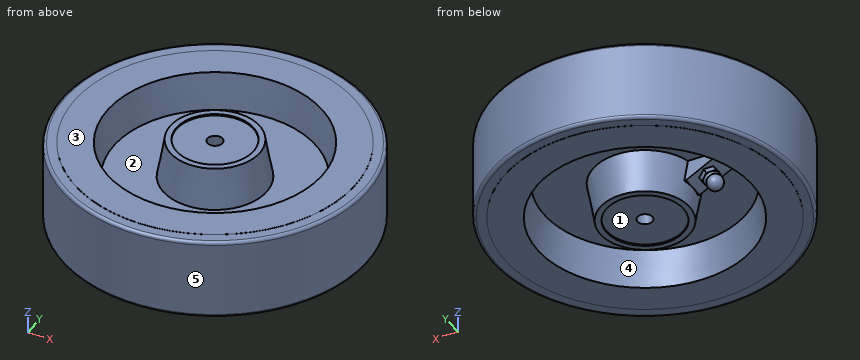
```python
from build123d import *

# Parameters (mm, degrees)
SKETCH1_R           = 150
SKETCH1_R_2         = 138
BOSS_EXTRUDE1_DEPTH = 40
FILLET4_R           = 3
BOSS_EXTRUDE2_DEPTH = 12.5
BOSS_EXTRUDE3_DEPTH = 5.5
SKETCH6_R           = 8.061337792
BOSS_EXTRUDE4_DEPTH = 3
BOSS_EXTRUDE4_TAPER = 30
SKETCH8_R           = 7.5
CUT_EXTRUDE1_DEPTH  = 229.714341483


with BuildPart() as part:
    # Sketch1 → Boss-Extrude1 (new, symmetric)
    with BuildSketch(Plane.XY):
        Circle(SKETCH1_R)
        Circle(SKETCH1_R_2, mode=Mode.SUBTRACT)
    extrude(amount=BOSS_EXTRUDE1_DEPTH, both=True)

    # Fillet4
    fillet4_edges = [part.edges().sort_by_distance(p)[0] for p in [
        (-150, 0, -40),
        (-150, 0, 40),
    ]]
    fillet(fillet4_edges, radius=FILLET4_R)



with BuildPart() as body_2:
    # Sketch3 → Revolve6 (revolve)
    with BuildSketch(Plane(origin=(0, 0, 0), x_dir=(1, 0, 0), z_dir=(0, 1, 0))):
        Polygon((0, -42), (0, 42), (-38, 42), (-38, 43.5), (-44, 43.5), (-50.920833993, 4.25), (-99.390952242, 4.25), (-105.718469789, 40.135135225), (-138, 40.135135225), (-138, 0.135135225), (-138, 0), (-138, -0.135135225), (-138, -40.135135225), (-105.718469789, -40.135135225), (-99.390952242, -4.25), (-50.920833993, -4.25), (-44, -43.5), (-38, -43.5), (-38, -42), align=None)
    revolve(axis=Axis((0, 0, -71.241325943), (0, 0, 1)))


with BuildPart() as part_1:
    add(part.part)

    add(body_2.part)  # Boss-Extrude2 merges body 2
    # Sketch4 → Boss-Extrude2 (add, symmetric)
    with BuildSketch(Plane(origin=(0, 0, 0), x_dir=(1, 0, 0), z_dir=(0, 1, 0))):
        Polygon((-44.394294379, 24.25), (-44.394294379, 4.25), (-79.394294379, 4.25), (-79.394294379, 7.25), (-47.394294379, 24.25), align=None)
    extrude(amount=BOSS_EXTRUDE2_DEPTH, both=True)

    # Sketch5 → Boss-Extrude3 (add)
    with BuildSketch(Plane(origin=(-20.479018336, 0, -38.548740398), x_dir=(-0.8831157194574107, 0, 0.46915522596174897), z_dir=(-0.46915522596174897, 0, -0.8831157194574107))):
        Polygon((56.704671627, -4.570014345), (56.607735872, 4.737911997), (48.498367326, 9.307926342), (40.485934534, 4.570014345), (40.582870289, -4.737911997), (48.692238836, -9.307926342), align=None)
    extrude(amount=BOSS_EXTRUDE3_DEPTH)

    # Sketch6 → Boss-Extrude4 (add)
    with BuildSketch(Plane(origin=(-23.059372079, 0, -43.405876855), x_dir=(-0.8831157194574104, 0, 0.46915522596174986), z_dir=(-0.4691552259617498, 0, -0.8831157194574103))):
        with Locations((48.595303081, 0)):
            Circle(SKETCH6_R)
    extrude(amount=BOSS_EXTRUDE4_DEPTH, taper=BOSS_EXTRUDE4_TAPER)

    # Sketch7 → Revolve7 (revolve)
    with BuildSketch(Plane(origin=(0, 0, 0), x_dir=(1, 0, 0), z_dir=(0, 1, 0)), mode=Mode.PRIVATE) as revolve7_sk:
        with BuildLine():
            ThreePointArc((-74.132927223, 32.5476045), (-66.020984278, 33.177231974), (-61.79262097, 26.225901681))
            Line((-61.79262097, 26.225901681), (-67.382113799, 23.256483615))
            Line((-67.382113799, 23.256483615), (-74.132927223, 32.5476045))
        make_face()
    revolve(revolve7_sk.sketch.rotate(Axis((-67.382113799, 0, -23.256483615), (-0.5878091288499389, 0, -0.8089996465021947)), 180), axis=Axis((-67.382113799, 0, -23.256483615), (-0.5878091288499389, 0, -0.8089996465021947)))

    # Sketch8 → Cut-Extrude1 (cut, through all)
    with BuildSketch(Plane(origin=(0, 0, -42), x_dir=(-1, 0, 0), z_dir=(0, 0, -1))):
        Circle(SKETCH8_R)
    extrude(amount=-CUT_EXTRUDE1_DEPTH, mode=Mode.SUBTRACT)


solid = part_1.part
```
Check sheet for the modelled part. Datum: model origin and axes. Units: mm. Face numbers are marked on the shaded views. A direction names the side the tool comes from. Round coordinates to 2 decimals unless told otherwise and drop trailing zeros. Loops run counter-clockwise (first coordinate to the right, second up) from the corner with the lowest first, then second, coordinate; pieces in that order, holes last. Notation, with made-up numbers: (12, 62.25) - (57, 62.25) arc R25 cw to (57, 98.25) - close; hole circle Ø2 at (14.25, -4.75). An arc over 180 degrees is marked (long way). Answer as a JSON object with one key per item and string values. Group by question number.
Q1. Set-up check for the marked faces 1 and 2: record each of +Z, -Z, +X, -X, +Y, -Y from which the full face is reachable in a straight line by a thin tool's end or side.
Q2. Gauge pin test, flat ends, axial feed: P1, Ø1, axis at x = -16, z = 10, coming from the +Y side; P2, Ø9, axis at x = 0, y = 0, coming from the +Z side; P3, Ø8, axis at x = -38, z = -6, coming from the +Y side; P4, Ø1, axis at x = -12, z = -12, coming from the +Y side. Record the tip position at first contact, or that the pin passes through.
Q3. Scan lines: line 1 along X through (y, z) = (40, -18.5); line 2 along Y through (x, z) = (-1.5, 18); line 3 along X through (y, z) = (-1, -23). Record each from-to range of solid material in increasing order. Write a range as [from, to].
Q4. Sectioned sample at A-A, the plane z = 9.5. Enter the section's corners in (x, y).
Q5. Mould release check, pull along Y, two halves, no side actions. Record for the marked faces 3, 4 and 5: released by +Y, released by -Y, zero draft, split by the parting line, or undercut.
Solution:
{
 "1": {"face 1": "-Z", "face 2": "+Z"},
 "2": {"P1": "stops at y = 149.2", "P2": "passes through", "P3": "stops at y = 146.1", "P4": "stops at y = 149.56"},
 "3": {"line 1": "x = [-144.57, -93.72], [-27.26, 27.26], [93.72, 144.57]", "line 2": "y = [-149.99, -101.8], [-48.47, -7.35], [7.35, 48.47], [101.8, 149.99]", "line 3": "x = [-150, -102.69], [-76.55, -58.13], [-49.75, -7.43], [7.43, 47.6], [102.69, 150]"},
 "4": {"outline": "circle Ø300 at (0, 0); circle Ø99.99 at (0, 0); hole circle Ø200.63 at (0, 0); hole circle Ø15 at (0, 0)"},
 "5": {"face 3": "zero draft", "face 4": "undercut", "face 5": "split by the parting line"}
}
